Geometry: final body of the model. Coordinates: model frame, mm. Face numbers are marked on the shaded views. A direction names the side the tool comes from. Coordinates: 2 decimals unless noted, no trailing zeros. Write each loop counter-clockwise with the first axis right and the second up, starting at its lowest first coordinate (ties: lowest second). Pieces come first, ordered by that corner, then holes.
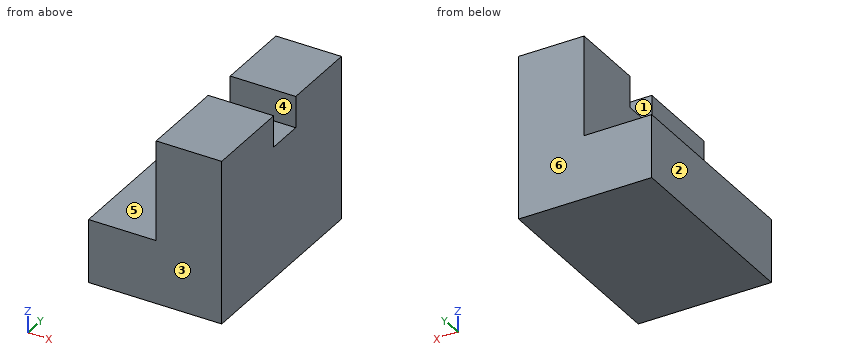
from build123d import *

# Parameters (mm, degrees)
F1_DEPTH = 38.1
F3_DEPTH = 12.7
F4_W     = 7.010136731
F4_H     = 5.9738913878
F5_DEPTH = 12.7


with BuildPart() as f1:
    # F0 (on Front) → F1 (new body)
    with BuildSketch(Plane.XZ):
        Polygon((0, 12.0385394319), (0, 0), (25.2677070918, 0), (25.2677070918, 31.0885394319), (12.8322897299, 31.0885394319), (12.8322897299, 12.0385394319), align=None)
    extrude(amount=F1_DEPTH)

    # F2 (on Right) → F3 (cut)
    with BuildSketch(Plane.YZ):
        Polygon((-12.249593623, 22.1733152866), (-12.249593623, 30.8565702289), (-24.6542412788, 31.1666876078), (-24.6542412788, 22.1733152866), align=None)
    extrude(amount=-F3_DEPTH, mode=Mode.SUBTRACT)

    # F4 (on face) → F5 (cut)
    with BuildSketch(Plane(origin=(12.8322897299, 0, 0), x_dir=(0, -1, 0), z_dir=(-1, 0, 0))):
        with Locations((18.044912722, 28.101593738)):
            Rectangle(F4_W, F4_H)
    extrude(amount=-F5_DEPTH, mode=Mode.SUBTRACT)


solid = f1.part
Item 1: Set-up query: the marked faces 5 and 6. Return all of +Z, -Z, +X, -X, +Y, -Y with unobstructed straight access to the full face (end or side cutting, diameter ignored); none if empty.
Derived:
face 5: +Z, -X, +Y, -Y
face 6: +Z, -Z, +X, -X, +Y
Item 2: Section D-D, the plane y = -19. Output: boundary loops of the cut face in (x, z), plus the area to 3 significant figures.
Derived:
outline: (0, 0) - (25.27, 0) - (25.27, 25.11) - (12.83, 25.11) - (12.83, 12.04) - (0, 12.04) - close
area: 467 mm2
Item 3: Pull-direction query (Y, two-part tool) for the marked faces 1, 2, 3 and 4; classes: released by +Y, released by -Y, zero draft, split by the parting line, or undercut.
Derived:
face 1: undercut
face 2: zero draft
face 3: released by -Y
face 4: undercut
Item 4: Section A-A, the plane x = 23. Output: boundary loops of the cut face in (y, z).
Derived:
outline: (-38.1, 0) - (0, 0) - (0, 31.09) - (-14.54, 31.09) - (-14.54, 25.11) - (-21.55, 25.11) - (-21.55, 31.09) - (-38.1, 31.09) - close
Item 5: Section B-B, the plane y = -31. Output: boundary loops of the cut face in (x, z).
Derived:
outline: (0, 0) - (25.27, 0) - (25.27, 31.09) - (12.83, 31.09) - (12.83, 12.04) - (0, 12.04) - close
Item 6: Section C-C, the plane z = 17.5. Output: boundary loops of the cut face in (x, y), plus the area to 3 significant figures.
Derived:
outline: (12.83, -38.1) - (25.27, -38.1) - (25.27, 0) - (12.83, 0) - close
area: 474 mm2
Item 7: Material intervals for probe 1 along X at (y, z) = (-15.5, 13); probe 2 along Z at (x, y) = (11.5, -32); probe 3 along Z at (x, y) = (24.25, -18.5), sorted ascending.
Derived:
probe 1: x = 12.83 to 25.27
probe 2: z = 0 to 12.04
probe 3: z = 0 to 25.11
Item 8: Pin query (flat end, axial travel): pin 1 (10.5 mm diameter, centred on x = 6.5, y = -17, fed in from +Z); pin 2 (8 mm diameter, centred on y = -14, z = 22, fed in from -X). Return the tip coordinate at first contact, or that it passes through.
Derived:
pin 1: stops at z = 12.04
pin 2: stops at x = 12.83
